Source: CAD feature listing. Evaluate the final solid. Frame: model axes, mm. A direction names the side the tool comes from. Round coordinates to 2 decimals unless told otherwise and drop trailing zeros. Loops run counter-clockwise (first coordinate to the right, second up) from the corner with the lowest first, then second, coordinate; pieces in that order, holes last. Notation, with made-up numbers: (-40, 77) - (-7, 77) arc R6 cw to (-7, 82) - close; hole circle Ø4 at (88, -12.75). An arc over 180 degrees is marked (long way). One line per question, with ' | ' between items.
from build123d import *

# Parameters (mm, degrees)
F2_W     = 200
F2_H     = 200
F2_R     = 82.6159275748
F2_R_2   = 75.2160474693
F3_DEPTH = 10
F4_R     = 4.99999


# Not quite as in the source:
# - a fillet or chamfer is up to 0.001 mm smaller than in the source, because OpenCascade refuses the exact size


with BuildPart() as f1:
    # F0 (on Front) → F1 (revolve)
    with BuildSketch(Plane.XZ):
        Polygon((-75, -75), (-10, 75), (-10, 80), (-13.2825942414, 80), (-82.6159275748, -80), (-75, -80), align=None)
    revolve(axis=Axis((0, 0, 2.9210224748), (0, 0, 1)))

    # F2 (on face) → F3 (join)
    with BuildSketch(Plane(origin=(0, 0, -80), x_dir=(1, 0, 0), z_dir=(0, 0, -1))):
        Rectangle(F2_W, F2_H)
        Circle(F2_R, mode=Mode.SUBTRACT)
        Circle(F2_R)
        Circle(F2_R_2, mode=Mode.SUBTRACT)
    extrude(amount=F3_DEPTH)

    # F4 (radius 5 in the source; OpenCascade refuses exactly that, so slightly less here)
    f4_edges = [f1.edges().sort_by_distance(p)[0] for p in [
        (-100, 100, -85),
        (100, 100, -85),
        (100, -100, -85),
        (-75.216047, 0, -90),
        (75, 0, -75),
        (-100, -100, -85),
        (0, 100, -90),
        (100, 0, -90),
        (0, -100, -90),
        (-100, 0, -90),
        (0, 100, -80),
        (-100, 0, -80),
        (100, 0, -80),
        (0, -100, -80),
        (82.615928, 0, -80),
        (13.282594, 0, 80),
        (10, 0, 75),
    ]]
    fillet(f4_edges, radius=F4_R)


solid = f1.part
1. Contact query for flat-ended pins moving along their axis: P1, Ø12, axis at x = -33.5, y = -58.5, coming from the -Z side; P2, Ø4, axis at x = 19, y = 30, coming from the +Z side; P3, Ø1, axis at x = 2, y = -25, coming from the +Z side. Output: stop coordinate, or through.
Worked out:
P1: stops at z = -71.34 | P2: stops at z = 33.32 | P3: stops at z = 53.93
2. Section query B-B, the plane z = 62. Return loops of the section in (x, y), plus the area to 3 significant figures.
Worked out:
outline: circle Ø42.17 at (0, 0); hole circle Ø31.27 at (0, 0) | area: 629 mm2
3. Section query A-A, the plane z = -31.5. Return loops of the section in (x, y).
Worked out:
outline: circle Ø123.2 at (0, 0); hole circle Ø112.3 at (0, 0)
4. Mould query, pull axis X, two halves, no side actions, for faces 4 (the cylindrical face through (98, -1, -89)), 5 (the cylindrical face through (-71.537, -22.528, -77.991)), 6 (the cylindrical face through (1, -99, -88)), 7 (the cylindrical face through (-9.54, -3, 78.05)). Classes: released by +X, released by -X, zero draft, split by the parting line, or undercut.
Worked out:
face 4: released by +X | face 5: undercut | face 6: zero draft | face 7: undercut
5. Access query for faces 1 (the flat face through (-86, -22, -80)), 2 (the cylindrical face through (71.743, -22.593, -82.465)), 3 (the cylindrical face through (98, -1, -81)). Directions: +Z, -Z, +X, -X, +Y, -Y. A direction counts if a zero-diameter tool reaches every point of the face in a straight line with its end or side. Return the directions, or none.
Worked out:
face 1: +Z | face 2: -Z | face 3: +Z, +X, +Y, -Y
6. Material intervals for probe 1 along X at (y, z) = (0, -77); probe 2 along Z at (x, y) = (84.5, 88); probe 3 along X at (y, z) = (-34, -51), sorted ascending.
Worked out:
probe 1: x = -81.32 to -75, 75 to 81.32 | probe 2: z = -90 to -80 | probe 3: x = -61.24 to -54.93, 54.93 to 61.24
